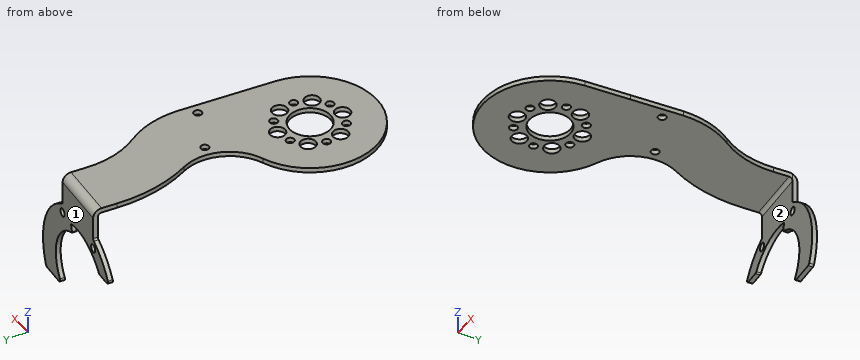
from build123d import *

# Parameters (mm, degrees)
EXTRUDE_1_DEPTH               = 2
EXTRUDE_2_DEPTH               = 2
HOLE_WIZARD_6_5_6_5_1_D       = 6.5
HOLE_WIZARD_6_5_6_5_1_DEPTH   = 51.1
HOLE_WIZARD_3_4_3_4_1_D       = 3.4
HOLE_WIZARD_3_4_3_4_1_DEPTH   = 51.1
HOLE_WIZARD_17_5_17_5_1_D     = 17.5
HOLE_WIZARD_17_5_17_5_1_DEPTH = 51.1
HOLE_WIZARD_3_4_3_4_2_D       = 3.4
HOLE_WIZARD_3_4_3_4_2_DEPTH   = 6.616402139
FILLET_1_R                    = 0.5
FILLET_2_R                    = 1
FILLET_3_R                    = 1.5
FILLET_4_R                    = 3.5


with BuildPart() as part:
    # 草图1 → 凸台-拉伸1 (new body)
    with BuildSketch(Plane.XY.offset(2)):
        with BuildLine():
            Line((19.991405474, 85.081394601), (20.688651416, 93.050952185))
            Line((20.688651416, 93.050952185), (-4.216216036, 95.229845754))
            Line((-4.216216036, 95.229845754), (-4.913461978, 87.260288169))
            ThreePointArc((-4.913461978, 87.260288169), (-4.101645556, 70.349808931), (1.198916656, 54.271021844))
            ThreePointArc((1.198916656, 54.271021844), (1.780962088, 38.051078797), (-9.859178165, 26.740355381))
            ThreePointArc((-9.859178165, 26.740355381), (-17.30251519, -22.646698835), (28.391548896, -2.483938668))
            Line((28.391548896, -2.483938668), (30.047508008, 16.443760595))
            Line((30.047508008, 16.443760595), (31.950173771, 38.33545379))
            ThreePointArc((31.950173771, 38.33545379), (30.780358309, 50.262124766), (25.93459204, 61.222621928))
            ThreePointArc((25.93459204, 61.222621928), (20.968028554, 72.655064005), (19.991405474, 85.081394601))
        make_face()
    extrude(amount=-EXTRUDE_1_DEPTH)

    # 草图2 → 凸台-拉伸2 (add)
    with BuildSketch(Plane(origin=(8.23621769, 94.14039897, 0), x_dir=(-0.9961946980917458, 0.08715574274765517, 0), z_dir=(0.08715574274765517, 0.9961946980917458, 0))):
        with BuildLine():
            Line((-15.491933385, -49.1), (-25.850531909, -49.1))
            ThreePointArc((-25.850531909, -49.1), (-26.858253967, -27.566679809), (-12.5, -11.48750305))
            Line((-12.5, -11.48750305), (-12.5, 2))
            Line((-12.5, 2), (12.5, 2))
            Line((12.5, 2), (12.5, -11.48750305))
            ThreePointArc((12.5, -11.48750305), (19.329574132, -16.156801489), (24.530313512, -22.590909091))
            ThreePointArc((24.530313512, -22.590909091), (24.538246516, -23.595433694), (23.669600757, -24.1))
            Line((23.669600757, -24.1), (17.437387992, -24.1))
            ThreePointArc((17.437387992, -24.1), (7.133948284, -16.553241572), (-5.629314231, -16.091113278))
            Line((-5.629314231, -16.091113278), (-4.658742812, -19.713335127))
            ThreePointArc((-4.658742812, -19.713335127), (-16.934605215, -30.999250357), (-14.67656847, -47.521052632))
            ThreePointArc((-14.67656847, -47.521052632), (-14.603410068, -48.558831468), (-15.491933385, -49.1))
        make_face()
    extrude(amount=EXTRUDE_2_DEPTH)

    # Ø6.5 (6.5) 直径孔1
    with Locations(Plane.XY.offset(2)):
        with Locations((11.058552598, -7.743281891), (1.176602527, 13.448628424), (-12.235155125, -5.705346533), (-11.058552598, 7.743281891), (12.235155125, 5.705346533), (-1.176602527, -13.448628424)):
            Hole(HOLE_WIZARD_6_5_6_5_1_D / 2, depth=HOLE_WIZARD_6_5_6_5_1_DEPTH)

    # Ø3.4 (3.4) 直径孔1
    with Locations(Plane.XY.offset(2)):
        with Locations((13.448628424, -1.176602527), (-5.705346533, 12.235155125), (-7.743281891, -11.058552598), (-13.448628424, 1.176602527), (7.743281891, 11.058552598), (5.705346534, -12.235155125), (26.9127025, 32.244479282), (7.366918218, 41.348863539)):
            Hole(HOLE_WIZARD_3_4_3_4_1_D / 2, depth=HOLE_WIZARD_3_4_3_4_1_DEPTH)

    # Ø17.5 (17.5) 直径孔1
    with Locations(Plane.XY.offset(2)):
        with Locations((0, 0)):
            Hole(HOLE_WIZARD_17_5_17_5_1_D / 2, depth=HOLE_WIZARD_17_5_17_5_1_DEPTH)

    # Ø3.4 (3.4) 直径孔2
    with Locations(Plane(origin=(8.23621769, 94.14039897, 0), x_dir=(0.9961946980917458, -0.08715574274765517, 0), z_dir=(-0.08715574274765517, -0.9961946980917458, 0))):
        with Locations((-25, 37.1), (-12.5, -15.449364905), (12.5, -15.449364905)):
            Hole(HOLE_WIZARD_3_4_3_4_2_D / 2, depth=HOLE_WIZARD_3_4_3_4_2_DEPTH)

    # 圆角1
    fillet_1_edges = [part.edges().sort_by_distance(p)[0] for p in [
        (12.964388321, 94.730557478, -19.713335127),
        (13.931266423, 94.645966605, -16.091113278),
    ]]
    fillet(fillet_1_edges, radius=FILLET_1_R)

    # 圆角2
    fillet_2_edges = [part.edges().sort_by_distance(p)[0] for p in [
        (-9.047660034, 96.65636217, -24.1),
        (-4.129060294, 96.226040452, -11.48750305),
        (20.775807159, 94.047146883, -11.48750305),
        (34.075536263, 92.883571359, -49.1),
    ]]
    fillet(fillet_2_edges, radius=FILLET_2_R)

    # 圆角3
    fillet_3_edges = [part.edges().sort_by_distance(p)[0] for p in [
        (8.23621769, 94.14039897, 0),
    ]]
    fillet(fillet_3_edges, radius=FILLET_3_R)

    # 圆角4
    fillet_4_edges = [part.edges().sort_by_distance(p)[0] for p in [
        (8.410529175, 96.132788366, 2),
    ]]
    fillet(fillet_4_edges, radius=FILLET_4_R)


solid = part.part
Source: CAD feature listing. Evaluate the final solid. Frame: model axes, mm. Face numbers are marked on the shaded views. A direction names the side the tool comes from. Give positions to 0.01 mm unless a question says otherwise; leave off trailing zeros. Write each loop counter-clockwise with the first axis right and the second up, starting at its lowest first coordinate (ties: lowest second). Pieces come first, ordered by that corner, then holes. Notation, with made-up numbers: M -31,19 L -19,19 A11 cw -19,24 Z; hole C -12,84 d2. An arc over 180 degrees is marked long. Return JSON: item names as keys, results as strings. Group by question number.
1) First-contact query: pin 1 Ø4.5 at (x, y) = (7.37, 41.35) entering from -Z; pin 2 Ø1.2 at (x, y) = (-14, 97.5) entering from -Z; pin 3 Ø5 at (x, z) = (-0.5, -17) entering from +Y. Flat tips, straight axial feed; report the tip coordinate or a pass-through.
2) Ray query, L1, parallel to Z at x = 3.5, y = 24; L2, parallel to Y at x = 33.5, z = -24.5; L3, parallel to Y at x = 1.5, z = -3. Return the intervals inside material, ascending.
3) Cut plane B-B, the plane y = 69.5. Output: boundary loops of the cut face in (x, z), then the cut area to 3 significant figures.
4) Cut plane A-A, the plane z = -29. Output: boundary loops of the cut face in (x, y), then the cut area to 3 significant figures.
5) Set-up query: the marked faces 1 and 2. Return all of +Z, -Z, +X, -X, +Y, -Y with unobstructed straight access to the full face (end or side cutting, diameter ignored); none if empty.
Data:
{
 "1": {"pin 1": "stops at z = 0", "pin 2": "stops at z = -24.1", "pin 3": "stops at y = 97.13"},
 "2": {"L1": "z = 0 to 2", "L2": "y = 91.93 to 93.94", "L3": "y = 94.73 to 96.74"},
 "3": {"outline": "M -3.94,0 L 21.9,0 L 21.9,2 L -3.94,2 Z", "area": "51.7 mm²"},
 "4": {"outline": "M 24.25,92.74 L 35.46,91.76 L 35.63,93.75 L 24.42,94.73 Z", "area": "22.5 mm²"},
 "5": {"face 1": "+Z, -Z, +X, +Y", "face 2": "-Z, -X, -Y"}
}
